Print and shaded views of the part. All mm, measured from the part's lowest x, y and z. A direction names the side the tool comes from. Round coordinates to 2 decimals unless told otherwise and drop trailing zeros. Loops run counter-clockwise (first coordinate to the right, second up) from the corner with the lowest first, then second, coordinate; pieces in that order, holes last. Notation, with made-up numbers: (12, 78) - (20, 78) arc R28 ccw to (20, 106) - close; hole circle Ø2 at (65, -1). An arc over 180 degrees is marked (long way). Answer as a JSON object with one key per item and string values.
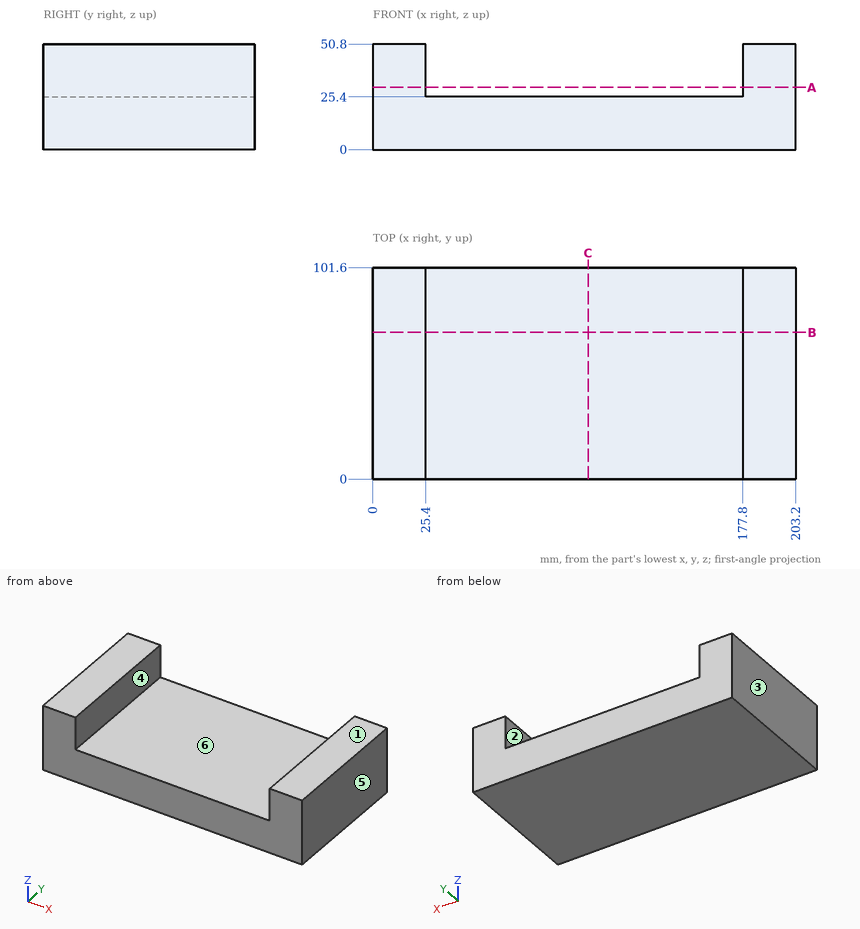
1) Slice it at A-A on z = 30. List the corners of the cut face in (x, y), then the cut area to 3 significant figures.
Values follow:
{"outline": "(0, 0) - (25.4, 0) - (25.4, 101.6) - (0, 101.6) - close; (177.8, 0) - (203.2, 0) - (203.2, 101.6) - (177.8, 101.6) - close", "area": "5,160 mm²"}
2) Tool access for the marked faces 5 and 6: list every direction of +Z, -Z, +X, -X, +Y, -Y with a clear straight run to the whole face (end or side of a thin tool).
Values follow:
{"face 5": "+Z, -Z, +X, +Y, -Y", "face 6": "+Z, +Y, -Y"}
3) Probe probe 1 along X at (y, z) = (27, 38); probe 2 along Z at (x, y) = (177.5, 51.5). List the from-to ranges inside material, lowest first.
Values follow:
{"probe 1": "0 to 25.4, 177.8 to 203.2", "probe 2": "0 to 25.4"}
4) Slice it at B-B on y = 70.5. List the corners of the cut face in (x, z), then the cut area to 3 significant figures.
Values follow:
{"outline": "(0, 0) - (203.2, 0) - (203.2, 50.8) - (177.8, 50.8) - (177.8, 25.4) - (25.4, 25.4) - (25.4, 50.8) - (0, 50.8) - close", "area": "6,450 mm²"}
5) Two-plate mould, pull along X, no slides. Class the marked faces 1, 2, 3 and 4: pulls with the +X half, pulls with the -X half, needs draft (parallel to the pull), parting line crosses it, or undercut.
Values follow:
{"face 1": "needs draft", "face 2": "undercut", "face 3": "pulls with the -X half", "face 4": "undercut"}
6) Slice it at C-C on x = 103.5. List the corners of the cut face in (y, z), then the cut area to 3 significant figures.
Values follow:
{"outline": "(0, 0) - (101.6, 0) - (101.6, 25.4) - (0, 25.4) - close", "area": "2,580 mm²"}
